Source: CAD feature listing. Evaluate the final solid. Frame: model axes, mm. Round coordinates to 2 decimals unless told otherwise and drop trailing zeros. Loops run counter-clockwise (first coordinate to the right, second up) from the corner with the lowest first, then second, coordinate; pieces in that order, holes last. Notation, with made-up numbers: M -11.5,-20.75 L -4.5,-20.75 A17 cw -4.5,-6.75 Z; hole C 13,35.25 d4. An arc over 180 degrees is marked long. One line per item, written item: value.
from build123d import *

# Parameters (mm, degrees)
SKETCH1_W           = 200
SKETCH1_H           = 10
BOSS_EXTRUDE1_DEPTH = 5
SKETCH2_R           = 1.9
CUT_EXTRUDE1_DEPTH  = 15


with BuildPart() as part:
    # Sketch1 → Boss-Extrude1 (new, symmetric)
    with BuildSketch(Plane.XY):
        Rectangle(SKETCH1_W, SKETCH1_H)
    extrude(amount=BOSS_EXTRUDE1_DEPTH, both=True)

    # Sketch2 → Cut-Extrude1 (cut, symmetric)
    with BuildSketch(Plane.XY):
        with Locations((-97.5, 0)):
            Circle(SKETCH2_R)
    extrude(amount=CUT_EXTRUDE1_DEPTH, both=True, mode=Mode.SUBTRACT)


solid = part.part
1. Pull-direction query (X, two-part tool) for faces 1 (the face through (100, 0, 0)), 2 (the face through (-100, 0, 0)), 3 (the face through (-1, -5, 0)), 4 (the face through (-99.4, 0.08, 0.07)); classes: released by +X, released by -X, zero draft, split by the parting line, or undercut.
Report:
face 1: released by +X
face 2: released by -X
face 3: zero draft
face 4: undercut
2. Section query A-A (x = -97.5). Return the cut outline in (y, z), and give its area (3 significant figures).
Report:
outline: M -5,-5 L -1.9,-5 L -1.9,5 L -5,5 Z; M 1.9,-5 L 5,-5 L 5,5 L 1.9,5 Z
area: 62.0 mm2
3. Ray query, line 1 (Y direction, x = -97.5, z = -2); line 2 (X direction, y = -1, z = -3.25). Return the intervals inside material, ascending. Write a range as [from, to].
Report:
line 1: y = [-5, -1.9], [1.9, 5]
line 2: x = [-100, -99.12], [-95.88, 100]
4. Section query B-B (y = 0). Return the cut outline in (x, z).
Report:
outline: M -100,-5 L -99.4,-5 L -99.4,5 L -100,5 Z; M -95.6,-5 L 100,-5 L 100,5 L -95.6,5 Z
